```python
from build123d import *

# Parameters (mm, degrees)
F2_DEPTH = 50
F0_R     = 9
F3_DEPTH = 41
F5_DEPTH = 150


# Not quite as in the source:
# - the dataset's text gives a spline's control points without its knots; the knots are read off the source's solid


with BuildPart() as f2:
    # F1 (on Front) → F2 (new body, symmetric)
    with BuildSketch(Plane.XZ):
        with BuildLine():
            ThreePointArc((-149.9588993892, 26.9134754342), (-154.8613095864, 26.2305586605), (-154.1783928127, 21.3281484633))
            add(Edge.make_bspline(
                [(-154.1783928127, 21.3281484633), (-125.9464059615, 0), (-3.9595449586, 0), (130.4603123693, 0), (151.5675187111, 0)],
                knots=[0, 0, 0, 0, 0.5033195654, 1, 1, 1, 1], degree=3))
            ThreePointArc((151.5675187111, 0), (155.0675187869, 3.5000000758), (151.5675187111, 7.0000001516))
            add(Edge.make_bspline(
                [(-149.9588993892, 26.9134754342), (-148.4478574546, 25.7719430693), (-145.1555512603, 23.5934371829), (-137.5039021405, 19.6641031988), (-126.0184700843, 15.5798750303), (-109.5578013858, 11.9753296087), (-90.8479253185, 9.5246754809), (-70.2937339258, 8.030291433), (-48.2800158692, 7.2686571064), (-29.0264464578, 7.0487772943), (-13.2581336189, 7.0012099028), (-1.291744917, 6.9996863373), (10.7653391732, 7.0000823662), (26.8484793874, 6.9999526881), (46.7909432723, 7.0000162503), (69.87873725, 6.9999959326), (98.7623960141, 7.0000025942), (129.847702251, 6.9999992634), (146.255449604, 7.0000001516), (151.5675187111, 7.0000001516)],
                knots=[0, 0, 0, 0, 0.03125, 0.0625, 0.125, 0.1875, 0.25, 0.3125, 0.375, 0.4375, 0.46875, 0.5, 0.53125, 0.5625, 0.625, 0.6875, 0.75, 0.875, 1, 1, 1, 1], degree=3))
        make_face()
    extrude(amount=F2_DEPTH, both=True)

    # F0 (on Top) → F3 (intersect)
    with BuildSketch(Plane.XY):
        with BuildLine():
            ThreePointArc((-150, 0), (-135.3553390593, -35.3553390593), (-100, -50))
            ThreePointArc((-100, -50), (-94.2011170994, -49.3098342645), (-88.4003291499, -48.635867795))
            ThreePointArc((-88.4003291499, -48.635867795), (-60.7572711034, -30.9839995602), (-50, 0))
            ThreePointArc((-50, 0), (-60.7572711034, 30.9839995602), (-88.4003291499, 48.635867795))
            ThreePointArc((-88.4003291499, 48.635867795), (-94.2011170994, 49.3098342645), (-100, 50))
            ThreePointArc((-100, 50), (-135.3553390593, 35.3553390593), (-150, 0))
        make_face()
        with Locations((-117.6522374153, 0)):
            Circle(F0_R, mode=Mode.SUBTRACT)
        with BuildLine():
            ThreePointArc((140.0476001587, -35.0236869248), (147.0878770301, -32.0780187539), (150, -25.0238002141))
            Line((150, -25.0238002141), (150, 0))
            Line((150, 0), (150, 25.0238002141))
            ThreePointArc((150, 25.0238002141), (147.0878770301, 32.0780187539), (140.0476001587, 35.0236869248))
            ThreePointArc((140.0476001587, 35.0236869248), (25.6372549098, 38.7018244409), (-88.4003291499, 48.635867795))
            ThreePointArc((-88.4003291499, 48.635867795), (-60.7572711034, 30.9839995602), (-50, 0))
            ThreePointArc((-50, 0), (-60.7572711034, -30.9839995602), (-88.4003291499, -48.635867795))
            ThreePointArc((-88.4003291499, -48.635867795), (25.6372549098, -38.7018244409), (140.0476001587, -35.0236869248))
        make_face()
    extrude(amount=F3_DEPTH, mode=Mode.INTERSECT)

    # F4 (on Right) → F5 (intersect, symmetric)
    with BuildSketch(Plane.YZ):
        with BuildLine():
            Line((-52.1002963765, 32.8564588929), (-55.3800071338, 3.0362728213))
            ThreePointArc((-55.3800071338, 3.0362728213), (0, 0), (55.3800071338, 3.0362728213))
            Line((55.3800071338, 3.0362728213), (52.1002963765, 32.8564588929))
            ThreePointArc((52.1002963765, 32.8564588929), (0, 30), (-52.1002963765, 32.8564588929))
        make_face()
    extrude(amount=F5_DEPTH, both=True, mode=Mode.INTERSECT)


solid = f2.part
```
The model under review builds one solid part; all positions refer to its coordinate system, in mm. Round coordinates to 2 decimals unless told otherwise and drop trailing zeros. Write each question's results on one line, items separated by ' | '. Start each with the question number.
Q1. Wall thickness on line 1 along Z through (x, y) = (-6, 6); line 2 along Z through (x, y) = (114, -7.5); line 3 along X through (y, z) = (-1, 20): over which ranges is each line inside the solid? List them lowest first. Write a range as [from, to].
Q2. Draft analysis for pull direction X (two halves, no side actions). For faces 1 (the cylindrical face through (-119.603, -8.786, 10.465)), 2 (the flat face through (150, 0, 3)), state which applies: pulls with the +X half, pulls with the -X half, needs draft (parallel to the pull), parting line crosses it, or undercut.
Q3. Insertion check: P1, Ø5, axis at x = 65.5, y = 28, coming from the -Z side; P2, Ø2, axis at x = 30, y = 23.5, coming from the -Z side; P3, Ø23.5, axis at x = -117.65, y = 0, coming from the +Z side; P4, Ø12, axis at y = -26, z = 6, coming from the +X side. Each pin has a flat end and moves straight along its axis. Give the tip position at first contact, or say it passes through.
Data:
1) line 1: z = [0.04, 7] | line 2: z = [0.06, 7] | line 3: x = [-149.99, -137.7]
2) face 1: undercut | face 2: pulls with the +X half
3) P1: stops at z = 0.64 | P2: stops at z = 0.5 | P3: stops at z = 16.94 | P4: stops at x = 150
